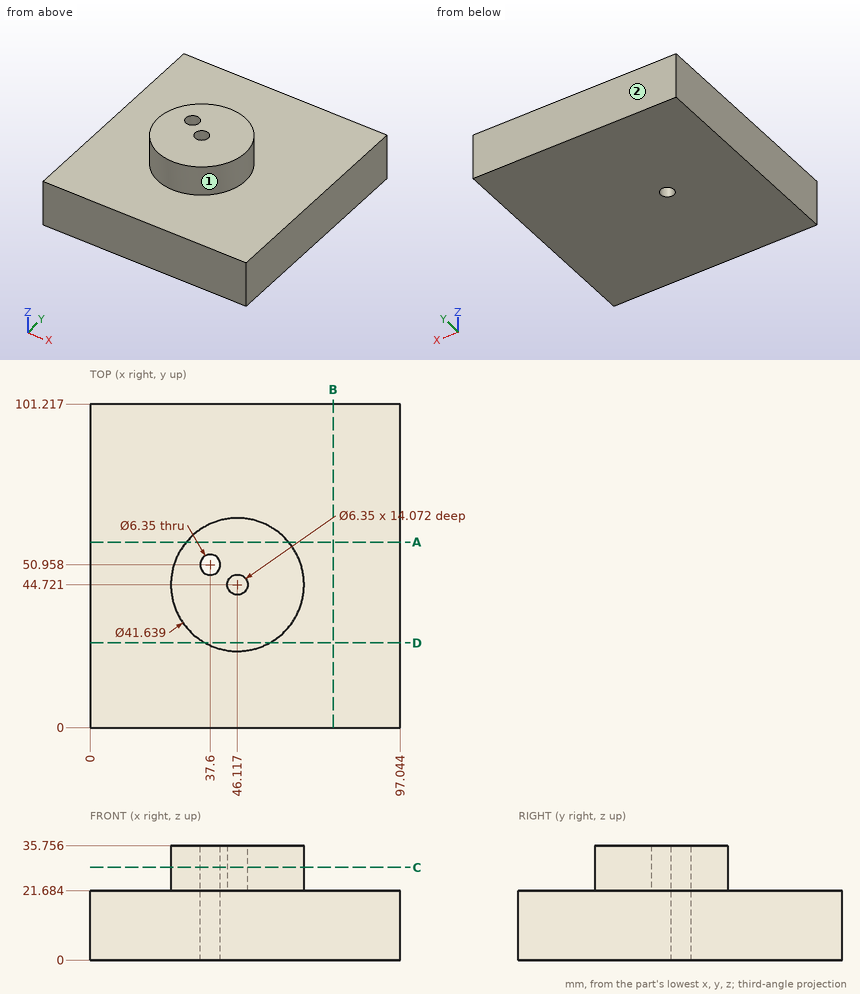
Answer from the drawing. Dimensions are ordinates in mm from the lowest x, y and z of the part. A direction names the side the tool comes from. Coordinates: 2 decimals unless noted, no trailing zeros. Loops run counter-clockwise (first coordinate to the right, second up) from the corner with the lowest first, then second, coordinate; pieces in that order, holes last.
1) Consider probe 1 along X at (y, z) = (51, 18.5) (1 decimal); probe 2 along Z at (x, y) = (11.5, 24); probe 3 along Y at (x, z) = (44.5, 33) (1 decimal). Determine where each line is inside the solid, lowest interval first.
Results:
probe 1: x = 0 to 34.4, 40.8 to 97
probe 2: z = 0 to 21.68
probe 3: y = 24 to 42, 47.5 to 65.5
2) Flat-ended cylindrical pins translate along their axes: pin 1 (8.5 mm diameter, centred on x = 37.6, y = 50.96, fed in from -Z); pin 2 (5.5 mm diameter, centred on x = 46.12, y = 44.72, fed in from +Z); pin 3 (1.5 mm diameter, centred on x = 56, z = 24.5, fed in from -Y). Find the tip coordinate at first contact, or state that the pin passes through.
Results:
pin 1: stops at z = 0
pin 2: stops at z = 21.68
pin 3: stops at y = 26.01
3) Section C-C (z = 29) is taken. Give the number of separate pieces and of enclosed holes in the cut face, plus the area to 3 significant figures.
Results:
separate pieces: 1
enclosed holes: 2
area: 1,300 mm2
4) Section A-A (y = 58) is taken. Give the vertices of the cut face in (x, z) (1 decimal), plus the area to 3 significant figures.
Results:
outline: (0, 0) - (97, 0) - (97, 21.7) - (62.2, 21.7) - (62.2, 35.8) - (30.1, 35.8) - (30.1, 21.7) - (0, 21.7) - close
area: 2,560 mm2
5) For the marked faces 1 and 2, determine the directions among +Z, -Z, +X, -X, +Y, -Y from which every point of the face is accessible in a straight line to the end or side of a thin tool.
Results:
face 1: +Z
face 2: +Z, -Z, +X, -X, +Y
6) Section D-D (y = 26.5) is taken. Give the vertices of the cut face in (x, z) (1 decimal).
Results:
outline: (0, 0) - (97, 0) - (97, 21.7) - (56.2, 21.7) - (56.2, 35.8) - (36, 35.8) - (36, 21.7) - (0, 21.7) - close
7) Section B-B (x = 76) is taken. Give the vertices of the cut face in (y, z).
Results:
outline: (0, 0) - (101.22, 0) - (101.22, 21.68) - (0, 21.68) - close
